For this review, take the finished solid that the model builds, in its own axes (mm). A direction names the side the tool comes from. Coordinates: 2 decimals unless noted, no trailing zeros. Loops run counter-clockwise (first coordinate to the right, second up) from the corner with the lowest first, then second, coordinate; pieces in that order, holes last. Notation, with made-up numbers: (7.5, 37.25) -> (34.5, 37.25) arc R24 cw to (34.5, 52.25) -> close; hole circle Ø11 at (34.5, 21.5). An arc over 180 degrees is marked (long way). Use a Markdown table: item, result.
from build123d import *

# Parameters (mm, degrees)
F0_R     = 10.5
F1_DEPTH = 10


with BuildPart() as f1:
    # F0 (on Front) → F1 (new body, symmetric)
    with BuildSketch(Plane.XZ):
        with BuildLine():
            ThreePointArc((12.649111, -3), (12.91198, -1.510225), (13, 0))
            ThreePointArc((13, 0), (12.91198, 1.510225), (12.649111, 3))
            ThreePointArc((12.649111, 3), (11.717824, 5.629617), (10.246951, 8))
            ThreePointArc((10.246951, 8), (-13, 0), (10.246951, -8))
            ThreePointArc((10.246951, -8), (11.717824, -5.629617), (12.649111, -3))
        make_face()
        Circle(F0_R, mode=Mode.SUBTRACT)
        with BuildLine():
            ThreePointArc((10.246951, 8), (11.717824, 5.629617), (12.649111, 3))
            Line((12.649111, 3), (78.205505, 3))
            ThreePointArc((78.205505, 3), (78.70852, 5.538311), (79.506098, 8))
            Line((79.506098, 8), (64.602166, 8))
            Line((64.602166, 8), (10.246951, 8))
        make_face()
        with BuildLine():
            Line((78.205505, -3), (12.649111, -3))
            ThreePointArc((12.649111, -3), (11.717824, -5.629617), (10.246951, -8))
            Line((10.246951, -8), (64.602166, -8))
            Line((64.602166, -8), (79.506098, -8))
            ThreePointArc((79.506098, -8), (78.70852, -5.538311), (78.205505, -3))
        make_face()
        with BuildLine():
            ThreePointArc((77.919916, 22.006825), (72.881564, 13.462612), (64.602166, 8))
            Line((64.602166, 8), (79.506098, 8))
            ThreePointArc((79.506098, 8), (104.070268, 21.620197), (122, 0))
            ThreePointArc((122, 0), (104.070268, -21.620197), (79.506098, -8))
            Line((79.506098, -8), (64.602166, -8))
            ThreePointArc((64.602166, -8), (72.881564, -13.462612), (77.919916, -22.006825))
            ThreePointArc((77.919916, -22.006825), (81.543964, -27.064374), (87.457159, -29))
            Line((87.457159, -29), (122, -29))
            Line((122, -29), (122, -25.805801))
            ThreePointArc((122, -25.805801), (122.220854, -24.676046), (122.850897, -23.712632))
            ThreePointArc((122.850897, -23.712632), (132.479081, -0.027734), (122.850897, 23.657163))
            ThreePointArc((122.850897, 23.657163), (122.220854, 24.620578), (122, 25.750333))
            Line((122, 25.750333), (122, 29))
            Line((122, 29), (87.457159, 29))
            ThreePointArc((87.457159, 29), (81.543964, 27.064374), (77.919916, 22.006825))
        make_face()
    extrude(amount=F1_DEPTH, both=True)


solid = f1.part
(1) Mouldability with a two-part tool opening along Z and no side actions: class faces 6 (the face through (10, 0.1, 3.2)), 7 (the face through (132.477, -0.14, -0.395)), 8 (the face through (76, -10, 4)) as pulls with the +Z half, pulls with the -Z half, needs draft (parallel to the pull), parting line crosses it, or undercut.
Found:
| item | result |
|---|---|
| face 6 | undercut |
| face 7 | parting line crosses it |
| face 8 | needs draft |
(2) For line 1 along Z through (x, y) = (0, 4.25); line 2 along Z through (x, y) = (17, 6.25); line 3 along X through (y, z) = (8.5, 3.5), list the stretches that pass through material, from the lowest coordinate up.
Found:
| item | result |
|---|---|
| line 1 | z = -13 to -10.5, 10.5 to 13 |
| line 2 | z = -8 to -3, 3 to 8 |
| line 3 | x = -12.52 to -9.9, 9.9 to 78.28, 121.72 to 132.3 |
(3) For pin 1 Ø6 at (x, y) = (24.5, 4) entering from +Z; pin 2 Ø5 at (y, z) = (-7, -18) entering from +X; pin 3 Ø2.5 at (y, z) = (2.5, 27.5) entering from +X, all flat-tipped, find the tip position at first contact; note any pin that passes through.
Found:
| item | result |
|---|---|
| pin 1 | stops at z = 8 |
| pin 2 | stops at x = 128.75 |
| pin 3 | stops at x = 122 |
(4) For faces 1 (the face through (78.718, -0.14, -5.573)), 2 (the face through (122, 0, -27)), 3 (the face through (38, 0, 8)), 4 (the face through (37, 0, -8)), 5 (the face through (122, 0, 27)), list the 3-axis set-ups (+Z, -Z, +X, -X, +Y, -Y) from which the entire face can be reached by the end or side of a thin tool; tool diameter is ignored.
Found:
| item | result |
|---|---|
| face 1 | +Y, -Y |
| face 2 | -Z, +X, +Y, -Y |
| face 3 | +Z, +Y, -Y |
| face 4 | -Z, +Y, -Y |
| face 5 | +Z, +X, +Y, -Y |
(5) Take a section at D-D on x = 83.5. Write out the cut boundary in (y, z).
Found:
| item | result |
|---|---|
| outline | (-10, -28.18) -> (10, -28.18) -> (10, -14.55) -> (-10, -14.55) -> close; (-10, 14.55) -> (10, 14.55) -> (10, 28.18) -> (-10, 28.18) -> close |
(6) Take a section at B-B on y = -2.5. Write out the cut boundary in (x, z), plus the area to 3 significant figures.
Found:
| item | result |
|---|---|
| outline | (10.25, -8) -> (64.6, -8) arc R22 cw to (77.92, -22.01) arc R10 ccw to (87.46, -29) -> (122, -29) -> (122, -25.81) arc R3 cw to (122.85, -23.71) arc R33.95 ccw to (122.85, 23.66) arc R3 cw to (122, 25.75) -> (122, 29) -> (87.46, 29) arc R10 ccw to (77.92, 22.01) arc R22 cw to (64.6, 8) -> (10.25, 8) arc R13 ccw (long way) to start; hole circle Ø21 at (0, 0); hole (12.65, -3) -> (78.21, -3) arc R22 ccw to (79.51, -8) arc R22 ccw (long way) to (79.51, 8) arc R22 ccw to (78.21, 3) -> (12.65, 3) arc R13 cw to (13, 0) arc R13 cw to start |
| area | 2,330 mm^2 |
(7) Take a section at C-C on z = -1.5. Write out the cut boundary in (x, y).
Found:
| item | result |
|---|---|
| outline | (-12.91, -10) -> (-10.39, -10) -> (-10.39, 10) -> (-12.91, 10) -> close; (10.39, -10) -> (12.91, -10) -> (12.91, 10) -> (10.39, 10) -> close; (121.95, -10) -> (132.45, -10) -> (132.45, 10) -> (121.95, 10) -> close |
(8) Take a section at A-A on x = 0. Write out the cut boundary in (y, z), plus the area to 3 significant figures.
Found:
| item | result |
|---|---|
| outline | (-10, -13) -> (10, -13) -> (10, -10.5) -> (-10, -10.5) -> close; (-10, 10.5) -> (10, 10.5) -> (10, 13) -> (-10, 13) -> close |
| area | 100 mm^2 |
